Check sheet for the modelled part. Datum: model origin and axes. Units: mm. A direction names the side the tool comes from. Round coordinates to 2 decimals unless told otherwise and drop trailing zeros. Order: outer loops, then holes, each group sorted by start corner. A loop starts at its lowest first (then second) coordinate and runs counter-clockwise, first axis right, second up.
(1) Depth check by flat-ended pin: pin 1 (1.5 mm diameter, centred on y = 6, z = -1, fed in from +X); pin 2 (2 mm diameter, centred on y = 4, z = 1.5, fed in from -X); pin 3 (3 mm diameter, centred on y = 3, z = 4.5, fed in from +X). Enter the tip coordinate at first touch or a pass-through.
(2) Sectioned sample at C-C, the plane y = 0.5. Enter the section's corners in (x, z), and give its area (3 significant figures).
(3) Thickness scan on probe 1 along Y at (x, z) = (-2.25, -1); probe 2 along Z at (x, y) = (0.5, 1.5); probe 3 along Z at (x, y) = (-0.5, 4.25). Record the ranges inside material, lowest first.
(4) Tool access check on faces 1 (the flat face through (-2.2, 2, 0.1)), 2 (the flat face through (0, 0, 0)). Record the directions out of +Z, -Z, +X, -X, +Y, -Y that give a thin tool (end or side, any length) a straight path to the whole face; none if there is none.
Autodesk Inventor part; units mm, degrees
ref_plane "YZ Plane" through (0, 0, 0) normal (1, 0, 0) x (0, 1, 0)
ref_plane "XZ Plane" through (0, 0, 0) normal (0, 1, 0) x (-1, 0, 0)
ref_plane "XY Plane" through (0, 0, 0) normal (0, 0, 1) x (1, 0, 0)
sketch "Sketch2" plane through (0, 0, 0) normal (0, 0, 1) x (1, 0, 0)
  line L0 (0, -1.6) -> (0, 9.6) construction
  line L1 (-7.2, 0) -> (1.2, 0) construction
  line L2 (0, 0) -> (-6, 0)
  line L3 (-6, 2) -> (-2, 2)
  line L4 (-2, 2) -> (-2, 4.114)
  line L5 (-2, 4.7135) -> (-2, 8)
  line L6 (-2, 8) -> (0, 8)
  line L7 (0, 0) -> (-6, 0)
  line L8 (-6, 2) -> (-6, 0)
  line L9 (-2, 3.3248) -> (-2, 5.5716)
  line L10 (0, 8) -> (0, 0)
  dimension "d0" = 2
  dimension "d1" = 6
  dimension "d3" = 2
  dimension "d4" = 8
revolve "Revolution1" add sketch "Sketch2" angle 360 about axis through (0, -10, 0) along (0, 1, 0)
chamfer "Chamfer1" distance 1 angle 45 1 edges at (6, 2, 0)
chamfer "Chamfer2" distance 1 angle 45 1 edges at (6, 0, 0)
properties part number "P006-Soupape_entree"
Derived:
1. pin 1: stops at x = 1.98
1. pin 2: stops at x = -1.94
1. pin 3: stops at x = 3.75
2. outline: circle Ø11 at (0, 0)
2. area: 95.1 mm2
3. probe 1: y = 0 to 2
3. probe 2: z = -5.48 to 5.48
3. probe 3: z = -1.94 to 1.94
4. face 1: +Y
4. face 2: +Z, -Z, +X, -X, -Y
